```python
from build123d import *

# Parameters (mm, degrees)
SKETCH_1_W                       = 186
SKETCH_1_H                       = 183
SKETCH_1_R                       = 20.5
SKETCH_1_R_2                     = 2.5
SKETCH_1_R_3                     = 2
SKETCH_1_R_4                     = 13
EXTRUDE_1_DEPTH                  = 5
SKETCH_2_W                       = 5
SKETCH_2_H                       = 20
EXTRUDE_2_DEPTH                  = 5
PATTERN_LINEAR_1_COUNT           = 5
PATTERN_LINEAR_1_PITCH           = 40
MIRROR_1_COPY_1_SKETCH_W         = 5
MIRROR_1_COPY_1_SKETCH_H         = 20
MIRROR_1_COPY_1_DEPTH            = 5
MIRROR_1_COPY_2_SKETCH_W         = 5
MIRROR_1_COPY_2_SKETCH_H         = 20
MIRROR_1_COPY_2_DEPTH            = 5
MIRROR_1_COPY_3_SKETCH_W         = 5
MIRROR_1_COPY_3_SKETCH_H         = 20
MIRROR_1_COPY_3_DEPTH            = 5
MIRROR_1_COPY_4_SKETCH_W         = 5
MIRROR_1_COPY_4_SKETCH_H         = 20
MIRROR_1_COPY_4_DEPTH            = 5
SKETCH_3_W                       = 20
SKETCH_3_H                       = 5
EXTRUDE_3_DEPTH                  = 5
PATTERN_LINEAR_2_COUNT           = 3
PATTERN_LINEAR_2_PITCH           = 40
PATTERN_LINEAR_3_COUNT           = 3
PATTERN_LINEAR_3_PITCH           = 40
SKETCH_4_W                       = 20
SKETCH_4_H                       = 10
EXTRUDE_4_DEPTH                  = 5
PATTERN_LINEAR_4_COUNT           = 3
PATTERN_LINEAR_4_PITCH           = 40
PATTERN_LINEAR_5_COPY_1_SKETCH_W = 20
PATTERN_LINEAR_5_COPY_1_SKETCH_H = 10
PATTERN_LINEAR_5_COPY_1_DEPTH    = 5
PATTERN_LINEAR_5_COPY_2_SKETCH_W = 20
PATTERN_LINEAR_5_COPY_2_SKETCH_H = 10
PATTERN_LINEAR_5_COPY_2_DEPTH    = 5
PATTERN_LINEAR_5_COPY_3_SKETCH_W = 20
PATTERN_LINEAR_5_COPY_3_SKETCH_H = 10
PATTERN_LINEAR_5_COPY_3_DEPTH    = 5
PATTERN_LINEAR_5_COPY_4_SKETCH_W = 20
PATTERN_LINEAR_5_COPY_4_SKETCH_H = 10
PATTERN_LINEAR_5_COPY_4_DEPTH    = 5
PATTERN_LINEAR_5_COPY_5_SKETCH_W = 20
PATTERN_LINEAR_5_COPY_5_SKETCH_H = 10
PATTERN_LINEAR_5_COPY_5_DEPTH    = 5
PATTERN_LINEAR_5_COPY_6_SKETCH_W = 20
PATTERN_LINEAR_5_COPY_6_SKETCH_H = 10
PATTERN_LINEAR_5_COPY_6_DEPTH    = 5
CUT_EXTRUDE_1_REACH              = 143.178
SKETCH_5_R                       = 2
PATTERN_LINEAR_6_COUNT           = 2
PATTERN_LINEAR_6_PITCH           = 80
PATTERN_LINEAR_7_COUNT           = 2
PATTERN_LINEAR_7_PITCH           = 80


with BuildPart() as part:
    # 스케치1 → 보스-돌출1 (new body)
    with BuildSketch(Plane.XY):
        Rectangle(SKETCH_1_W, SKETCH_1_H)
        with Locations((-35.25, -28.5)):
            Circle(SKETCH_1_R, mode=Mode.SUBTRACT)
        with Locations((-61.25, -28.5)):
            Circle(SKETCH_1_R_2, mode=Mode.SUBTRACT)
        with Locations(Location((-9.25, -28.5, 0), (0, 0, 180))):
            Circle(SKETCH_1_R_2, mode=Mode.SUBTRACT)
        with Locations((35.221625496, -30.5)):
            Circle(SKETCH_1_R, mode=Mode.SUBTRACT)
        with Locations((16.836849185, -12.115223689)):
            Circle(SKETCH_1_R_2, mode=Mode.SUBTRACT)
        with Locations((53.606401807, -48.884776311)):
            Circle(SKETCH_1_R_2, mode=Mode.SUBTRACT)
        with Locations((39.42261881, 19)):
            Circle(SKETCH_1_R_3, mode=Mode.SUBTRACT)
        with Locations((39.42261881, 36.5)):
            Circle(SKETCH_1_R_4, mode=Mode.SUBTRACT)
        with Locations((21.92261881, 36.5)):
            Circle(SKETCH_1_R_3, mode=Mode.SUBTRACT)
        with Locations((39.42261881, 54)):
            Circle(SKETCH_1_R_3, mode=Mode.SUBTRACT)
        with Locations((56.92261881, 36.5)):
            Circle(SKETCH_1_R_3, mode=Mode.SUBTRACT)
    extrude(amount=EXTRUDE_1_DEPTH)

    # 스케치2 → 보스-돌출2 (add)
    with BuildSketch(Plane.XY.offset(5)):
        with Locations((-95.5, -81.5)):
            Rectangle(SKETCH_2_W, SKETCH_2_H)
    extrude_2 = extrude(amount=-EXTRUDE_2_DEPTH)

    # 선형 패턴1: 보스-돌출2 ×5
    with Locations(*[(0, i * PATTERN_LINEAR_1_PITCH, 0) for i in range(1, PATTERN_LINEAR_1_COUNT)]):
        add(extrude_2)

    # 대칭 복사1: 보스-돌출2 across plane
    add(extrude_2.mirror(Plane(origin=(0, 0, 0), x_dir=(0, 0, 1), z_dir=(1, 0, 0))))

    # 대칭 복사1 copy 1 sketch → 대칭 복사1 copy 1 (add)
    with BuildSketch(Plane(origin=(0, 40, 5), x_dir=(-1, 0, 0), z_dir=(0, 0, 1))):
        with Locations((-95.5, 81.5)):
            Rectangle(MIRROR_1_COPY_1_SKETCH_W, MIRROR_1_COPY_1_SKETCH_H)
    extrude(amount=-MIRROR_1_COPY_1_DEPTH)

    # 대칭 복사1 copy 2 sketch → 대칭 복사1 copy 2 (add)
    with BuildSketch(Plane(origin=(0, 80, 5), x_dir=(-1, 0, 0), z_dir=(0, 0, 1))):
        with Locations((-95.5, 81.5)):
            Rectangle(MIRROR_1_COPY_2_SKETCH_W, MIRROR_1_COPY_2_SKETCH_H)
    extrude(amount=-MIRROR_1_COPY_2_DEPTH)

    # 대칭 복사1 copy 3 sketch → 대칭 복사1 copy 3 (add)
    with BuildSketch(Plane(origin=(0, 120, 5), x_dir=(-1, 0, 0), z_dir=(0, 0, 1))):
        with Locations((-95.5, 81.5)):
            Rectangle(MIRROR_1_COPY_3_SKETCH_W, MIRROR_1_COPY_3_SKETCH_H)
    extrude(amount=-MIRROR_1_COPY_3_DEPTH)

    # 대칭 복사1 copy 4 sketch → 대칭 복사1 copy 4 (add)
    with BuildSketch(Plane(origin=(0, 160, 5), x_dir=(-1, 0, 0), z_dir=(0, 0, 1))):
        with Locations((-95.5, 81.5)):
            Rectangle(MIRROR_1_COPY_4_SKETCH_W, MIRROR_1_COPY_4_SKETCH_H)
    extrude(amount=-MIRROR_1_COPY_4_DEPTH)

    # 스케치3 → 보스-돌출3 (add)
    with BuildSketch(Plane.XY.offset(5)):
        with Locations((0, 94)):
            Rectangle(SKETCH_3_W, SKETCH_3_H)
    extrude_3 = extrude(amount=-EXTRUDE_3_DEPTH)

    # 선형 패턴2: 보스-돌출3 ×3
    with Locations(*[(i * PATTERN_LINEAR_2_PITCH, 0, 0) for i in range(1, PATTERN_LINEAR_2_COUNT)]):
        add(extrude_3)

    # 선형 패턴3: 보스-돌출3 ×3
    with Locations(*[(-i * PATTERN_LINEAR_3_PITCH, 0, 0) for i in range(1, PATTERN_LINEAR_3_COUNT)]):
        add(extrude_3)

    # 스케치4 → 보스-돌출4 (add)
    with BuildSketch(Plane.XY.offset(5)):
        with Locations((0, -96.5)):
            Rectangle(SKETCH_4_W, SKETCH_4_H)
    extrude_4 = extrude(amount=-EXTRUDE_4_DEPTH)

    # 선형 패턴4: 보스-돌출4 ×3
    with Locations(*[(i * PATTERN_LINEAR_4_PITCH, 0, 0) for i in range(1, PATTERN_LINEAR_4_COUNT)]):
        add(extrude_4)

    # 선형 패턴5 copy 1 sketch → 선형 패턴5 copy 1 (add)
    with BuildSketch(Plane.XY.offset(5)):
        with Locations((0, -96.5)):
            Rectangle(PATTERN_LINEAR_5_COPY_1_SKETCH_W, PATTERN_LINEAR_5_COPY_1_SKETCH_H)
    extrude(amount=-PATTERN_LINEAR_5_COPY_1_DEPTH)

    # 선형 패턴5 copy 2 sketch → 선형 패턴5 copy 2 (add)
    with BuildSketch(Plane(origin=(-40, 0, 5), x_dir=(1, 0, 0), z_dir=(0, 0, 1))):
        with Locations((0, -96.5)):
            Rectangle(PATTERN_LINEAR_5_COPY_2_SKETCH_W, PATTERN_LINEAR_5_COPY_2_SKETCH_H)
    extrude(amount=-PATTERN_LINEAR_5_COPY_2_DEPTH)

    # 선형 패턴5 copy 3 sketch → 선형 패턴5 copy 3 (add)
    with BuildSketch(Plane(origin=(40, 0, 5), x_dir=(1, 0, 0), z_dir=(0, 0, 1))):
        with Locations((0, -96.5)):
            Rectangle(PATTERN_LINEAR_5_COPY_3_SKETCH_W, PATTERN_LINEAR_5_COPY_3_SKETCH_H)
    extrude(amount=-PATTERN_LINEAR_5_COPY_3_DEPTH)

    # 선형 패턴5 copy 4 sketch → 선형 패턴5 copy 4 (add)
    with BuildSketch(Plane.XY.offset(5)):
        with Locations((0, -96.5)):
            Rectangle(PATTERN_LINEAR_5_COPY_4_SKETCH_W, PATTERN_LINEAR_5_COPY_4_SKETCH_H)
    extrude(amount=-PATTERN_LINEAR_5_COPY_4_DEPTH)

    # 선형 패턴5 copy 5 sketch → 선형 패턴5 copy 5 (add)
    with BuildSketch(Plane(origin=(-40, 0, 5), x_dir=(1, 0, 0), z_dir=(0, 0, 1))):
        with Locations((0, -96.5)):
            Rectangle(PATTERN_LINEAR_5_COPY_5_SKETCH_W, PATTERN_LINEAR_5_COPY_5_SKETCH_H)
    extrude(amount=-PATTERN_LINEAR_5_COPY_5_DEPTH)

    # 선형 패턴5 copy 6 sketch → 선형 패턴5 copy 6 (add)
    with BuildSketch(Plane(origin=(-80, 0, 5), x_dir=(1, 0, 0), z_dir=(0, 0, 1))):
        with Locations((0, -96.5)):
            Rectangle(PATTERN_LINEAR_5_COPY_6_SKETCH_W, PATTERN_LINEAR_5_COPY_6_SKETCH_H)
    extrude(amount=-PATTERN_LINEAR_5_COPY_6_DEPTH)

    # 스케치5 → 컷-돌출1 (cut, up to next)
    with BuildSketch(Plane(origin=(0, 0, 0), x_dir=(-1, 0, 0), z_dir=(0, 0, -1)), mode=Mode.PRIVATE) as cut_extrude_1_sk1:
        with Locations((0, -85.2)):
            Circle(SKETCH_5_R)
    cut_extrude_1_tool1 = extrude(cut_extrude_1_sk1.sketch, amount=-CUT_EXTRUDE_1_REACH, mode=Mode.PRIVATE) & part.part
    cut_extrude_1 = cut_extrude_1_tool1.solids().sort_by_distance((0, -85.2, 0))[0]
    add(cut_extrude_1, mode=Mode.SUBTRACT)

    # 선형 패턴6: 컷-돌출1 ×2
    with Locations(*[(i * PATTERN_LINEAR_6_PITCH, 0, 0) for i in range(1, PATTERN_LINEAR_6_COUNT)]):
        add(cut_extrude_1, mode=Mode.SUBTRACT)

    # 선형 패턴7: 컷-돌출1 ×2
    with Locations(*[(-i * PATTERN_LINEAR_7_PITCH, 0, 0) for i in range(1, PATTERN_LINEAR_7_COUNT)]):
        add(cut_extrude_1, mode=Mode.SUBTRACT)


solid = part.part
```
Model file for the job. Use its own axes, mm. A direction names the side the tool comes from. Round coordinates to 2 decimals unless told otherwise and drop trailing zeros. Order: outer loops, then holes, each group sorted by start corner. A loop starts at its lowest first (then second) coordinate and runs counter-clockwise, first axis right, second up. Notation, with made-up numbers: (-36.5, 44) -> (20.5, 44) arc R20 ccw to (20.5, 59) -> close; hole circle Ø9 at (11, 7). An arc over 180 degrees is marked (long way). Use one line per item in the form item = value.
Item 1: Cut at D-D, the plane z = 0.95. Give the number of separate pieces and of enclosed holes in the cut face, and give its area (3 significant figures).
Returned:
separate_pieces = 1
enclosed_holes = 14
area = 33,200 mm^2
Item 2: Tool access for faces 1 (the face through (93, 18, 2)), 2 (the face through (10, -97, 3)), 3 (the face through (-96, 28.5, 3)), 4 (the face through (10, 94, 3)): list every direction of +Z, -Z, +X, -X, +Y, -Y with a clear straight run to the whole face (end or side of a thin tool).
Returned:
face_1 = +Z, -Z, +X
face_2 = +Z, -Z, -Y
face_3 = +Z, -Z, -X
face_4 = +Z, -Z, +Y
Item 3: Cut at C-C, the plane x = 47. Write the cut outline in (y, z).
Returned:
outline = (-101.5, 0) -> (-47.28, 0) -> (-47.28, 5) -> (-101.5, 5) -> close; (-13.72, 0) -> (25.94, 0) -> (25.94, 5) -> (-13.72, 5) -> close; (47.06, 0) -> (96.5, 0) -> (96.5, 5) -> (47.06, 5) -> close
Item 4: Flat gauge pins, fed straight in: pin 1 Ø2.5 at (x, y) = (56.92, 36.5) entering from -Z; pin 2 Ø1.5 at (y, z) = (-62.5, 2.5) entering from +X; pin 3 Ø1.5 at (x, z) = (-95.5, 3) entering from +Y; pin 4 Ø2.5 at (y, z) = (-99, 2.5) entering from -X. Where does each tip first touch, or does it go through?
Returned:
pin_1 = through
pin_2 = 93
pin_3 = 88.5
pin_4 = -90
Item 5: Cut at A-A, the plane x = -35.25. Write the cut outline in (y, z), and give its area (3 significant figures).
Returned:
outline = (-101.5, 0) -> (-49, 0) -> (-49, 5) -> (-101.5, 5) -> close; (-8, 0) -> (96.5, 0) -> (96.5, 5) -> (-8, 5) -> close
area = 785 mm^2
Item 6: Drill centre lines: line 1 (Y direction, x = 45, z = 1.45); line 2 (Y direction, x = -61.25, z = 3.7); line 3 (X direction, y = -42, z = 3.3). Where is each one in solid material? Low to high.
Returned:
line_1 = -101.5 to -48.52, -12.48 to 24.76, 48.24 to 96.5
line_2 = -91.5 to -31, -26 to 91.5
line_3 = -98 to -50.68, -19.82 to 18.25, 52.19 to 98
Item 7: Cut at B-B, the plane x = -61.25. Write the cut outline in (y, z).
Returned:
outline = (-91.5, 0) -> (-31, 0) -> (-31, 5) -> (-91.5, 5) -> close; (-26, 0) -> (91.5, 0) -> (91.5, 5) -> (-26, 5) -> close
Item 8: Pull direction X, two halves, no side cores. Call faces 5 (the face through (98, 79, 3)), 6 (the face through (-60, -91.5, 3)), 7 (the face through (96, -31.5, 3)), 8 (the face through (-93, -22, 2)): released by +X, released by -X, zero draft, split by the parting line, or undercut.
Returned:
face_5 = released by +X
face_6 = undercut
face_7 = zero draft
face_8 = released by -X
